For this review, take the finished solid that the model builds, in its own axes (mm). Face numbers are marked on the shaded views. A direction names the side the tool comes from. Give positions to 0.01 mm unless a question says otherwise; leave off trailing zeros. Write each loop counter-clockwise with the first axis right and the second up, starting at its lowest first coordinate (ties: lowest second). Pieces come first, ordered by that corner, then holes.
1) Wall thickness on line 1 along Z through (x, y) = (0, 3.5); line 2 along Y through (x, z) = (0, -8); line 3 along Y through (x, z) = (-4.5, 4): over which ranges is each line inside the solid? List them lowest first.
2) We need section A-A on x = 0. Give the boundary of the cut face in (y, z).
3) Draft analysis for pull direction Y (two halves, no side actions). For the marked faces 1, 2, 3 and 4, state which applies: pulls with the +Y half, pulls with the -Y half, needs draft (parallel to the pull), parting line crosses it, or undercut.
4) We need section C-C on x = -30.5. Give the boundary of the cut face in (y, z), and give its area (3 significant figures).
5) We need section B-B on z = -9.75. Give the boundary of the cut face in (x, y) (3 decimals).
6) We need section D-D on y = 7.5. Give the boundary of the cut face in (x, z), and give its area (3 significant figures).
7) Machinability: for the marked faces 5, 6, 7 and 8, which of the approach directions +Z, -Z, +X, -X, +Y, -Y give a long, thin tool a straight path to every point of the face, cutting with its end or side? Answer none if there is none.
8) For P1, Ø16, axis at x = -53.213, y = 19.05, coming from the -Z side; P2, Ø6, axis at x = 0, y = 16, coming from the +Z side; P3, Ø5.5, axis at x = 0, z = 3.175, coming from the +Y side, all flat-tipped, find the tip position at first contact; note any pin that passes through.
from build123d import *

# Parameters (mm, degrees)
SKETCH1_W           = 20.066
SKETCH1_H           = 25.4
BOSS_EXTRUDE1_DEPTH = 6.35
SKETCH2_W           = 20.066
SKETCH2_H           = 25.4
BOSS_EXTRUDE2_DEPTH = 6.35
SKETCH3_W           = 25.4
SKETCH3_H           = 38.1
BOSS_EXTRUDE3_DEPTH = 6.35
SKETCH4_W           = 50.8
SKETCH4_H           = 38.1
BOSS_EXTRUDE4_DEPTH = 6.35
SKETCH6_R           = 2.286
CUT_EXTRUDE1_DEPTH  = 7.35
SKETCH7_R           = 2.286
CUT_EXTRUDE2_DEPTH  = 7.35
SKETCH8_R           = 6.1595
SKETCH8_R_2         = 3.175
CUT_EXTRUDE3_DEPTH  = 26.4
FILLET1_R           = 6.35


with BuildPart() as part:
    # Sketch1 → Boss-Extrude1 (new body)
    with BuildSketch(Plane(origin=(0, 0, 0), x_dir=(1, 0, 0), z_dir=(0, 1, 0))):
        Rectangle(SKETCH1_W, SKETCH1_H)
    extrude(amount=BOSS_EXTRUDE1_DEPTH)

    # Sketch2 → Boss-Extrude2 (add)
    with BuildSketch(Plane(origin=(0, 0, -12.7), x_dir=(-1, 0, 0), z_dir=(0, 0, -1))):
        with Locations((0, 12.7)):
            Rectangle(SKETCH2_W, SKETCH2_H)
    extrude(amount=-BOSS_EXTRUDE2_DEPTH)

    # Sketch3 → Boss-Extrude3 (add)
    with BuildSketch(Plane.ZY.offset(10.033)):
        with Locations((0, 19.05)):
            Rectangle(SKETCH3_W, SKETCH3_H)
    extrude(amount=BOSS_EXTRUDE3_DEPTH)

    # Sketch4 → Boss-Extrude4 (add)
    with BuildSketch(Plane.XY.offset(12.7)):
        with Locations((-41.783, 19.05)):
            Rectangle(SKETCH4_W, SKETCH4_H)
    extrude(amount=-BOSS_EXTRUDE4_DEPTH)

    # Sketch6 → Cut-Extrude1 (cut, through all)
    with BuildSketch(Plane.XY.offset(-6.35)):
        with Locations((0, 15.875)):
            Circle(SKETCH6_R)
    extrude(amount=-CUT_EXTRUDE1_DEPTH, mode=Mode.SUBTRACT)

    # Sketch7 → Cut-Extrude2 (cut, through all)
    with BuildSketch(Plane(origin=(0, 6.35, 0), x_dir=(1, 0, 0), z_dir=(0, 1, 0))):
        with Locations((0, -3.175)):
            Circle(SKETCH7_R)
    extrude(amount=-CUT_EXTRUDE2_DEPTH, mode=Mode.SUBTRACT)

    # Sketch8 → Cut-Extrude3 (cut, through all)
    with BuildSketch(Plane.XY.offset(12.7)):
        with Locations((-53.213, 19.05)):
            Circle(SKETCH8_R)
        with Locations((-29.083, 19.05)):
            Circle(SKETCH8_R_2)
    extrude(amount=-CUT_EXTRUDE3_DEPTH, mode=Mode.SUBTRACT)

    # Fillet1
    fillet1_edges = [part.edges().sort_by_distance(p)[0] for p in [
        (-10.033, 25.4, -9.525),
        (10.033, 25.4, -9.525),
        (-10.033, 22.225, 12.7),
        (-16.383, 19.05, 6.35),
        (-67.183, 0, 9.525),
        (-67.183, 38.1, 9.525),
        (10.033, 3.175, 12.7),
    ]]
    fillet(fillet1_edges, radius=FILLET1_R)


solid = part.part
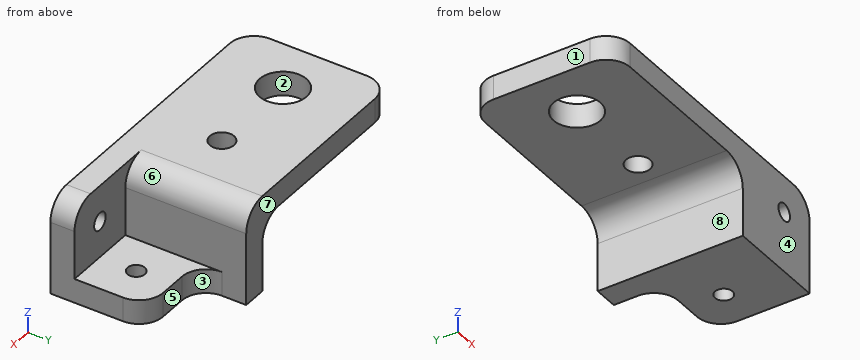
Results list:
1. line 1: z = -12.7 to 0.89, 5.46 to 12.7
1. line 2: y = 0 to 13.59, 18.16 to 25.4
1. line 3: y = 0 to 6.35
2. outline: (0, -12.7) - (13.59, -12.7) - (13.59, -6.35) - (6.35, -6.35) - (6.35, 0.89) - (0, 0.89) - close; (0, 5.46) - (6.35, 5.46) - (6.35, 12.7) - (0, 12.7) - close; (18.16, -12.7) - (25.4, -12.7) - (25.4, -6.35) - (18.16, -6.35) - close
3. face 1: needs draft
3. face 2: undercut
3. face 3: pulls with the +Y half
3. face 4: pulls with the -Y half
4. outline: (0, 6.35) - (16.21, 6.35) - (16.21, 12.7) - (0, 12.7) - close; (21.89, 6.35) - (38.1, 6.35) - (38.1, 12.7) - (21.89, 12.7) - close
4. area: 206 mm2
5. outline: (-16.383, 0) - (10.033, 0) - (10.033, 19.05) arc R6.35 ccw to (3.683, 25.4) - (-3.683, 25.4) arc R6.35 cw to (-10.033, 31.75) - (-10.033, 38.1) - (-16.383, 38.1) - close; hole circle Ø4.572 at (0, 15.875)
6. outline: (-67.18, 6.35) - (-22.73, 6.35) arc R6.35 cw to (-16.38, 0) - (-16.38, -12.7) - (10.03, -12.7) - (10.03, -6.35) - (-10.03, -6.35) - (-10.03, 6.35) arc R6.35 ccw to (-16.38, 12.7) - (-67.18, 12.7) - close
6. area: 611 mm2
7. face 5: +Z, -Z, +X, +Y
7. face 6: +Z, +X, +Y
7. face 7: +Z, -Z, +X, -X, +Y
7. face 8: -Z, -X, +Y, -Y
8. P1: stops at z = 6.35
8. P2: stops at z = -6.35
8. P3: stops at y = 6.35
